Check sheet for the modelled part. Datum: model origin and axes. Units: mm. Face numbers are marked on the shaded views. A direction names the side the tool comes from. Round coordinates to 2 decimals unless told otherwise and drop trailing zeros. Write each loop counter-clockwise with the first axis right and the second up, starting at its lowest first coordinate (ties: lowest second). Pieces come first, ordered by that corner, then holes. Notation, with made-up numbers: M -16,-20.5 L -10,-20.5 A31 cw -10,16.5 Z; hole C 71,64.5 d8. An arc over 180 degrees is marked long. Put each result on its own line as item: value.
Autodesk Inventor part; units mm, degrees
ref_plane "YZ Plane" through (0, 0, 0) normal (1, 0, 0) x (0, 1, 0)
ref_plane "XZ Plane" through (0, 0, 0) normal (0, 1, 0) x (-1, 0, 0)
ref_plane "XY Plane" through (0, 0, 0) normal (0, 0, 1) x (1, 0, 0)
sketch "Boceto1" plane through (0, 0, 0) normal (1, 0, 0) x (0, 1, 0)
  line L0 (10, 16.4587) -> (10, -17.5667)
  line L1 (10, -17.5667) -> (7.5667, -20)
  line L2 (7.5667, -20) -> (-5.3553, -20)
  line L3 (-5.3553, -20) -> (-10, -15.3553)
  line L4 (-10, -15.3553) -> (-10, 14.7117)
  line L5 (-10, 14.7117) -> (-4.7117, 20)
  line L6 (-4.7117, 20) -> (6.4587, 20)
  line L7 (6.4587, 20) -> (10, 16.4587)
  line L8 (0, 0) -> (31.525, 0) construction
  line L9 (0, 0) -> (0, -54.6434) construction
  dimension "d0" = 135
  dimension "d2" = 135
  dimension "d3" = 135
  dimension "d5" = 40
  dimension "d6" = 20
extrude "Extrusión1" add sketch "Boceto1" along normal mid plane 3
sketch "Boceto2" plane through (0, 0, 0) normal (0, 1, 0) x (-1, 0, 0)
  line L0 (0, 0) -> (-24, 0) construction
  line L1 (1.5, -25) -> (-23.8963, -25)
  line L2 (-23.8963, -25) -> (-36.5, -7)
  line L3 (-36.5, -7) -> (-36.5, 7)
  line L4 (-36.5, 7) -> (-23.8963, 25)
  line L5 (-23.8963, 25) -> (1.5, 25)
  line L6 (-1.5, 20) -> (1.5, 20)
  line L7 (-1.5, -15.3553) -> (-1.5, -20)
  line L8 (-1.5, 20) -> (-1.5, -20)
  line L9 (1.5, 20) -> (-1.5, 20)
  line L10 (1.5, -20) -> (1.5, -15.3553)
  line L11 (1.5, -20) -> (-1.5, -20)
  line L12 (1.5, -20) -> (-1.5, -20)
  line L13 (1.5, -20) -> (1.5, -25)
  line L14 (1.5, 20) -> (1.5, 25)
  line L15 (1.5, 16.4587) -> (1.5, -17.5667)
  line L16 (-10.5, 19) -> (-23, 19)
  line L17 (-23, 19) -> (-23, -5)
  line L18 (-23, -5) -> (-10.5, -5)
  line L19 (-10.5, -5) -> (-10.5, 19)
  line L20 (-10.5, 7) -> (-23, 7) construction
  circle A0 centre (-7.5, 7) radius 1.5
  circle A1 centre (-26, 7) radius 1.5
  circle A2 centre (-16.75, -12) radius 1.5
  line L21 (-16.75, -5) -> (-16.75, -34) construction
  dimension "d9" = 50
  dimension "d10" = 38
  dimension "d11" = 145
  dimension "d12" = 145
  dimension "d13" = 12.5
  dimension "d14" = 24
  dimension "d15" = 6
  dimension "d16" = 12
  dimension "d17" = 3
  dimension "d18" = 3
  dimension "d19" = 3
  dimension "d20" = 3
  dimension "d21" = 3
  dimension "d22" = 7
extrude "Extrusión2" add sketch "Boceto2" along normal mid plane 3
sketch "Boceto3" plane through (0, 0, 0) normal (0, 1, 0) x (-1, 0, 0)
  line L0 (-36.5, -8) -> (-29.5, -8)
  line L1 (-29.5, -8) -> (-29.5, 8)
  line L2 (-29.5, 8) -> (-36.5, 8)
  line L3 (-36.5, 8) -> (-36.5, -8)
  line L4 (0, 0) -> (-66, 0) construction
  point P0 (-33, -8)
  point P1 (-33, 8)
  dimension "d25" = 7
  dimension "d34" = 8
  dimension "d35" = 8
extrude "Extrusión3" add sketch "Boceto3" along normal mid plane 9
sketch "Boceto4" plane through (0, 4.5, 0) normal (0, 1, 0) x (1, 0, 0)
  circle A0 centre (33, 5.5) radius 1.5
  circle A1 centre (33, -5.5) radius 1.5
  line L0 (-1.5, 15.3553) -> (-1.5, -14.7117)
  line L1 (-1.5, 0) -> (97, 0) construction
  line L2 (97, 0) -> (96, 0)
  point P0 (0, 0)
  dimension "d28" = 3
  dimension "d29" = 3
  dimension "d30" = 11
  dimension "d31" = 5.5
extrude "Extrusión4" cut sketch "Boceto4" against normal up to surface (9 mm away)
sketch "Boceto5" plane through (-1.5, 0, 0) normal (-1, 0, 0) x (0, 0, 1)
  circle A0 centre (0, 0) radius 3.5
  dimension "d38" = 7
extrude "Extrusión5" cut sketch "Boceto5" against normal blind 1
equation "\"Radio_pliegue\" = Grosor"
equation "\"Anchura_desahogo_plegado\" = Grosor"
equation "\"Profundidad_desahogo_plegado\" = 0.5 * Grosor"
equation "\"Tamaño_destalonado\" = 4 * Grosor"
equation "\"Remanente_mínimo\" = 2 * Grosor"
equation "\"Radiodetransición\" = Radio_pliegue"
equation "\"Tamaño_de_radio_de_Jacobi\" = Radio_pliegue"
equation "\"TamañoSeparación\" = Grosor"
properties part number "Pinza_pieza1"
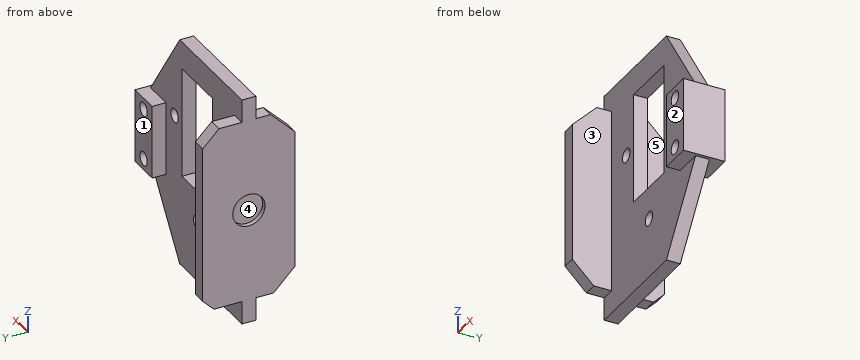
1. Access from +Z, -Z, +X, -X, +Y, -Y to the whole of each face (thin tool, end or side, straight path). Record for the marked faces 1, 2 and 3.
Computed values:
face 1: +Z, -Z, +X, +Y
face 2: +Z, -Z, +X, -Y
face 3: +Z, -Z, -Y
2. Cross-section at B-B (y = -2.5). Enter the section's corners in (x, z).
Computed values:
outline: M -1.5,-20 L 1.5,-20 L 1.5,20 L -1.5,20 L -1.5,2.45 L -0.5,2.45 L -0.5,-2.45 L -1.5,-2.45 Z; M 29.5,-8 L 36.5,-8 L 36.5,8 L 29.5,8 Z; hole C 33,-5.5 d3; hole C 33,5.5 d3
3. Cross-section at D-D (y = 0). Enter the section's corners in (x, z).
Computed values:
outline: M -1.5,-25 L 23.9,-25 L 35.8,-8 L 36.5,-8 L 36.5,8 L 35.8,8 L 23.9,25 L -1.5,25 L -1.5,3.5 L -0.5,3.5 L -0.5,-3.5 L -1.5,-3.5 Z; hole C 7.5,7 d3; hole M 10.5,-5 L 23,-5 L 23,19 L 10.5,19 Z; hole C 16.75,-12 d3; hole C 26,7 d3; hole C 33,-5.5 d3; hole C 33,5.5 d3
4. Scan lines: probe 1 along X at (y, z) = (0, -5.5); probe 2 along Z at (x, y) = (7.5, 0.2); probe 3 along X at (y, z) = (-2.25, -3). Record each from-to range of solid material in increasing order.
Computed values:
probe 1: x = -1.5 to 31.5, 34.5 to 36.5
probe 2: z = -25 to 5.5, 8.5 to 25
probe 3: x = -1.5 to 1.5, 29.5 to 36.5
5. Depth check by flat-ended pin: pin 1 Ø7.5 at (x, z) = (33, 2.5) entering from +Y; pin 2 Ø5 at (x, z) = (8.5, -19) entering from -Y; pin 3 Ø0.9 at (x, y) = (0, 6) entering from -Z; pin 4 Ø18.5 at (x, z) = (10, -4) entering from +Y. Enter the tip coordinate at first touch or a pass-through.
Computed values:
pin 1: stops at y = 4.5
pin 2: stops at y = -1.5
pin 3: stops at z = -20
pin 4: stops at y = 10
6. Cross-section at A-A (x = 7.5). Enter the section's corners in (y, z).
Computed values:
outline: M -1.5,-25 L 1.5,-25 L 1.5,5.5 L -1.5,5.5 Z; M -1.5,8.5 L 1.5,8.5 L 1.5,25 L -1.5,25 Z
7. Cross-section at C-C (z = 0). Enter the section's corners in (x, y), then the cut area to 4 significant figures.
Computed values:
outline: M -1.5,-10 L 1.5,-10 L 1.5,-1.5 L 10.5,-1.5 L 10.5,1.5 L 1.5,1.5 L 1.5,10 L -1.5,10 L -1.5,3.5 L -0.5,3.5 L -0.5,-3.5 L -1.5,-3.5 Z; M 23,-1.5 L 29.5,-1.5 L 29.5,-4.5 L 36.5,-4.5 L 36.5,4.5 L 29.5,4.5 L 29.5,1.5 L 23,1.5 Z
area: 162.5 mm2
8. Release check for a two-part mould opening along Z. For the marked faces 4 and 5 record: +Z half, -Z half, draft (parallel to the pull), parting line (faces both ways), or undercut.
Computed values:
face 4: undercut
face 5: draft
